Autodesk Inventor part; units mm, degrees
ref_plane "YZ Plane" through (0, 0, 0) normal (1, 0, 0) x (0, 1, 0)
ref_plane "XZ Plane" through (0, 0, 0) normal (0, 1, 0) x (-1, 0, 0)
ref_plane "XY Plane" through (0, 0, 0) normal (0, 0, 1) x (1, 0, 0)
sketch "Sketch3" plane through (0, 0, 0) normal (0, 1, 0) x (-1, 0, 0)
  line L0 (0, 0) -> (35, 0)
  line L1 (35, 0) -> (35, -24)
  line L2 (35, -24) -> (0, -24)
  line L3 (0, -24) -> (0, 0)
  dimension "d7" = 35
  dimension "d8" = 24
extrude "Extrusion2" add sketch "Sketch3" along normal blind 23
sketch "Sketch4" plane through (0, 0, 0) normal (0, -1, 0) x (1, 0, 0)
  line L0 (-35, 0) -> (0, 0)
  line L1 (-35, 0) -> (0, 0)
  line L2 (-35, -24) -> (-35, 0)
  line L3 (-35, -12) -> (-17.5, -12)
  line L4 (-35, -21) -> (0, -21)
  line L5 (0, -21) -> (0, -3)
  line L6 (0, -3) -> (-35, -3)
  line L7 (-35, -3) -> (-35, -21)
  line L8 (-35, -21) -> (0, -3) construction
  line L9 (0, -21) -> (-35, -3) construction
  dimension "d11" = 35
  dimension "d12" = 18
extrude "Extrusion3" cut sketch "Sketch4" against normal blind 20
sketch "Sketch5" plane through (0, 0, -24) normal (1, 0, 0) x (0, 0, -1)
  line L0 (-21, 0) -> (-24, 0)
  line L1 (0, 0) -> (0, 23)
  line L2 (-24, 0) -> (0, 0)
  line L3 (0, 0) -> (0, 1)
  line L4 (0, 1) -> (-24, 1)
  line L5 (-24, 1) -> (-24, 0)
  dimension "d15" = 1
extrude "Extrusion4" cut sketch "Sketch5" against normal blind 50.1625
sketch "Sketch6" plane through (-35, 23, -24) normal (-1, 0, 0) x (0, 0, 1)
  line L0 (3, -22) -> (0, -22)
  line L1 (0, -22) -> (3, -22)
  line L2 (3, -22) -> (3, -3)
  line L3 (3, -3) -> (0, -3)
  line L4 (0, -3) -> (0, -22)
  line L5 (24, 0) -> (0, 0)
  line L6 (0, -3) -> (24, -3)
  line L7 (24, -3) -> (24, 0)
  line L8 (24, 0) -> (0, 0)
  line L9 (0, 0) -> (0, -3)
  line L10 (24, -22) -> (24, 0)
  line L11 (21, -22) -> (21, -3)
  line L12 (24, 0) -> (21, 0)
  line L13 (21, 0) -> (21, -22)
  line L14 (21, -22) -> (24, -22)
  line L15 (24, -22) -> (24, 0)
  point P0 (24, -23)
extrude "Extrusion5" add sketch "Sketch6" along normal blind 15
sketch "Sketch7" plane through (-50, 23, -24) normal (-1, 0, 0) x (0, 0, 1)
  line L0 (24, 0) -> (0, 0)
  line L1 (12, 0) -> (12, -22)
  line L2 (0, 0) -> (0, -22)
  line L3 (0, 0) -> (24, 0)
  line L4 (0, -22) -> (3, -22)
  line L5 (21, -22) -> (24, -22)
  line L6 (0, -22) -> (24, -22)
  point P0 (24, -23)
sketch "Sketch8" plane through (-50, 23, -24) normal (-1, 0, 0) x (0, 0, 1)
  line L0 (0, -22) -> (3, -22)
  line L1 (21, -3) -> (21, -22)
  line L2 (3, -22) -> (21, -22)
  line L3 (21, -22) -> (21, -19)
  line L4 (21, -19) -> (3, -19)
  line L5 (3, -19) -> (3, -22)
  point P0 (24, -23)
  dimension "d20" = 3
extrude "Extrusion6" add sketch "Sketch8" against normal up to surface (50 mm away)
sketch "Sketch9" plane through (0, 23, 0) normal (1, 0, 0) x (0, 0, -1)
  line L0 (3, -19) -> (3, -3)
  line L1 (0, 0) -> (24, 0)
  line L2 (3, -3) -> (21, -3)
  line L3 (21, -3) -> (21, 0)
  line L4 (21, 0) -> (3, 0)
  line L5 (3, 0) -> (3, -3)
  point P0 (0, -23)
  point P1 (3, 0)
  dimension "d23" = 18
extrude "Extrusion7" cut sketch "Sketch9" against normal up to surface (50 mm away)
sketch "Sketch10" plane through (0, 1, -24) normal (0, 0, -1) x (-1, 0, 0)
  line L0 (50, 22) -> (50, 3)
  line L1 (50, 22) -> (47, 22)
  line L2 (0, 22) -> (50, 22)
  line L3 (47, 22) -> (31, 22)
  line L4 (31, 22) -> (31, 9.5)
  line L5 (31, 9.5) -> (47, 9.5)
  line L6 (47, 9.5) -> (47, 22)
  point P0 (0, -1)
  dimension "d26" = 3
  dimension "d27" = 16
  dimension "d28" = 12.5
extrude "Extrusion8" cut sketch "Sketch10" against normal blind 30.6375
sketch "Sketch12" plane through (0, 1, -24) normal (0, 0, -1) x (-1, 0, 0)
  line L0 (31, 9.5) -> (47, 9.5)
  line L1 (47, 9.5) -> (39, 9.5)
  line L2 (39, 9.5) -> (39, 0)
  line L3 (50, 0) -> (0, 0)
  line L4 (36, 4) -> (42, 4)
  line L5 (42, 4) -> (42, -4)
  line L6 (42, -4) -> (36, -4)
  line L7 (36, -4) -> (36, 4)
  line L8 (36, 4) -> (42, -4) construction
  line L9 (42, 4) -> (36, -4) construction
  line L10 (42, 4) -> (44, 4)
  line L11 (44, 4) -> (44, 0)
  line L12 (44, 0) -> (42, 0)
  line L13 (42, 0) -> (42, 4)
  line L14 (36, 4) -> (34, 4)
  line L15 (34, 4) -> (34, 0)
  line L16 (34, 0) -> (36, 0)
  line L17 (36, 0) -> (36, 4)
  point P0 (0, -1)
  dimension "d34" = 6
  dimension "d35" = 8
  dimension "d36" = 2
  dimension "d37" = 2
extrude "Extrusion10" cut sketch "Sketch12" against normal up to surface (24 mm away) contours L4 L5 L3 L2 | L2 L3 L7 L4 | L7 L3 L15 L14 | L10 L11 L3 L5
properties part number "batteryContainer"
Here's how the part is built. I have some questions about the finished solid (model axes, mm). A direction names the side the tool comes from. Give positions to 0.01 mm unless a question says otherwise; leave off trailing zeros. Order: outer loops, then holes, each group sorted by start corner. A loop starts at its lowest first (then second) coordinate and runs counter-clockwise, first axis right, second up. Notation, with made-up numbers: M -15.75,-8 L 28.25,-8 A16 cw 28.25,1 Z; hole C 0.5,38 d5. An arc over 180 degrees is marked long. Answer as a JSON object with one key per item and string values. Group by question number.
1) Suppose I cut it at D-D, the plane x = -13.5. Write out the boundary of the cut face in (y, z).
2) Suppose I cut it at A-A, the plane z = -19.25. Write out the boundary of the cut face in (x, y), plus the area to 3 significant figures.
3) We'd pull the mould along Z, two halves only. Please class faces 6 (the flat face through (-31, 17, -23)), 7 (the flat face through (-17, 4, -12)), 8 (the flat face through (-19, 12, 0)): pulls with the +Z half, pulls with the -Z half, needs draft (parallel to the pull), parting line crosses it, or undercut.
4) I'm going to push flat-ended pins straight in: pin 1 Ø6.5 at (x, z) = (-47.5, -13.5) entering from +Y; pin 2 Ø2.5 at (x, z) = (-40, -2) entering from +Y; pin 3 Ø1.5 at (x, z) = (-40.5, -23) entering from -Y. Where does each tip first touch, or does it pass through?
5) On a 3-axis mill with a long thin cutter (end or side, diameter ignored), from which of +Z, -Z, +X, -X, +Y, -Y can I reach the whole of each face in a straight line? I mean faces 1 (the flat face through (-44, 3, -12)), 2 (the flat face through (-19, 13, -3)), 3 (the flat face through (-20, 12, -24)), 4 (the flat face through (-31, 17, -2)), 5 (the flat face through (-17, 1, -12)). Say none if no direction works.
6) Suppose I cut it at B-B, the plane x = -31.5. Write out the boundary of the cut face in (y, z), plus the area to 3 significant figures.
7) Suppose I cut it at C-C, the plane y = 14.25. Write out the boundary of the cut face in (x, z).
8) Please list where these lines run through material, in increasing order: L1, parallel to Z at x = -29, y = 15.5; L2, parallel to Y at x = -23.5, z = -3.75; L3, parallel to X at y = 2.5, z = -7.25. Write a range as [from, to].
Results found:
{
 "1": {"outline": "M 1,-24 L 23,-24 L 23,-21 L 4,-21 L 4,-3 L 23,-3 L 23,0 L 1,0 Z"},
 "2": {"outline": "M -50,1 L -44,1 L -44,4 L -50,4 Z; M -34,1 L 0,1 L 0,4 L -34,4 Z", "area": "120 mm²"},
 "3": {"face 6": "needs draft", "face 7": "undercut", "face 8": "pulls with the +Z half"},
 "4": {"pin 1": "y = 4", "pin 2": "y = 10.5", "pin 3": "y = 5"},
 "5": {"face 1": "+Z, -Z, -Y", "face 2": "+X, -X, +Y", "face 3": "-Z, +X, -X, +Y, -Y", "face 4": "+Z, -Z, +Y", "face 5": "+Z, -Z, +X, -X, -Y"},
 "6": {"outline": "M 1,-24 L 10.5,-24 L 10.5,-21 L 4,-21 L 4,-3 L 10.5,-3 L 10.5,0 L 1,0 Z", "area": "111 mm²"},
 "7": {"outline": "M -50,-24 L -47,-24 L -47,-21 L -50,-21 Z; M -50,-3 L -47,-3 L -47,0 L -50,0 Z; M -31,-24 L 0,-24 L 0,-21 L -31,-21 Z; M -31,-3 L 0,-3 L 0,0 L -31,0 Z"},
 "8": {"L1": "[-24, -21], [-3, 0]", "L2": "[1, 4]", "L3": "[-50, -44], [-34, 0]"}
}
